The figure shows three views and two pictorial views of one solid part (mm, origin at its lowest corner). Answer the questions. A direction names the side the tool comes from. Coordinates: 2 decimals unless noted, no trailing zeros. Order: outer loops, then holes, each group sorted by start corner. A loop starts at its lowest first (then second) coordinate and runs counter-clockwise, first axis right, second up. Notation, with made-up numbers: (10, 41.25) - (68, 41.25) arc R27 cw to (68, 71.25) - close; hole circle Ø3 at (69, -14.5). An arc over 180 degrees is marked (long way). Use one line per item in the form item = value. Start each with the question number.
Item 1: A tool of negligible diameter and unlimited length cuts with its end or side. For the marked faces 1 and 2, from which of +Z, -Z, +X, -X, +Y, -Y can it reach the whole face along a straight path? Write none if from no direction.
Item 2: Section C-C, the plane z = 1 is taken. Write down the section's boundary in (x, y), and give its area (3 significant figures).
Item 3: Each of these flat-tipped pins is pushed along its axis until it touches: pin 1 Ø4.5 at (x, z) = (9.5, 7) entering from -Y; pin 2 Ø0.7 at (x, y) = (12, 9) entering from +Z; pin 3 Ø3 at (x, z) = (29.5, 7) entering from +Y; pin 4 Ø1 at (x, y) = (12, 8.5) entering from -Z. Where does it stop, or does it pass through?
Item 4: Section D-D, the plane y = 2.5 is taken. Write down the section's boundary in (x, z), and give its area (3 significant figures).
Item 5: The mould has two halves that part along Z. Classify the marked faces 3, 4 and 5: released by +Z, released by -Z, zero draft, split by the parting line, or undercut.
Item 6: Consider line 1 along X through (y, z) = (7.3, 7); line 2 along X through (y, z) = (5, 6); line 3 along Z through (x, y) = (9.5, 6.45). Determine where each line is inside the solid, lowest interval first. Write a range as [from, to].
Item 7: Section B-B, the plane x = 9.5 is taken. Write down the section's boundary in (y, z), and give its area (3 significant figures).
Item 8: Section A-A, the plane z = 7 is taken. Write down the section's boundary in (x, y).
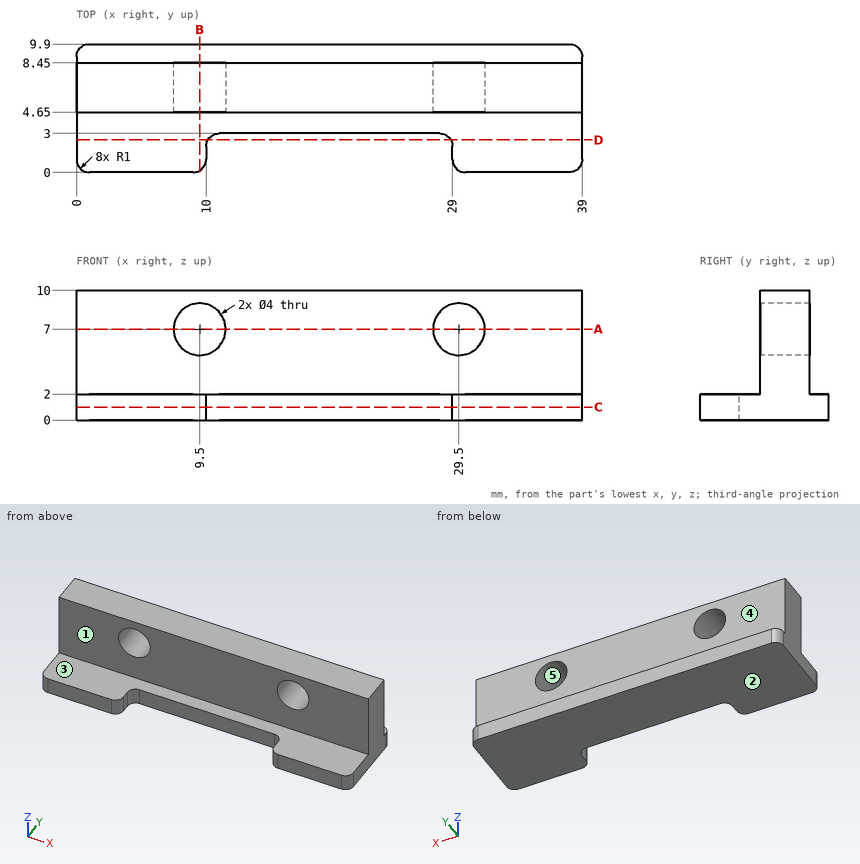
Response:
q1.face_1 = +Z, +X, -X, -Y
q1.face_2 = -Z, +X, -X, +Y, -Y
q2.outline = (0, 1) arc R1 ccw to (1, 0) - (9, 0) arc R1 ccw to (10, 1) - (10, 2) arc R1 cw to (11, 3) - (28, 3) arc R1 cw to (29, 2) - (29, 1) arc R1 ccw to (30, 0) - (38, 0) arc R1 ccw to (39, 1) - (39, 8.9) arc R1 ccw to (38, 9.9) - (1, 9.9) arc R1 ccw to (0, 8.9) - close
q2.area = 328 mm2
q3.pin_1 = 4.65
q3.pin_2 = 2
q3.pin_3 = through
q3.pin_4 = 0
q4.outline = (0, 0) - (10.13, 0) - (10.13, 2) - (0, 2) - close; (28.87, 0) - (39, 0) - (39, 2) - (28.87, 2) - close
q4.area = 40.5 mm2
q5.face_3 = released by +Z
q5.face_4 = zero draft
q5.face_5 = undercut
q6.line_1 = [0, 7.5], [11.5, 27.5], [31.5, 39]
q6.line_2 = [0, 7.77], [11.23, 27.77], [31.23, 39]
q6.line_3 = [0, 5], [9, 10]
q7.outline = (0.13, 0) - (9.9, 0) - (9.9, 2) - (8.45, 2) - (8.45, 5) - (4.65, 5) - (4.65, 2) - (0.13, 2) - close; (4.65, 9) - (8.45, 9) - (8.45, 10) - (4.65, 10) - close
q7.area = 34.7 mm2
q8.outline = (0, 4.65) - (7.5, 4.65) - (7.5, 8.45) - (0, 8.45) - close; (11.5, 4.65) - (27.5, 4.65) - (27.5, 8.45) - (11.5, 8.45) - close; (31.5, 4.65) - (39, 4.65) - (39, 8.45) - (31.5, 8.45) - close
